Source: CAD feature listing. Evaluate the final solid. Frame: model axes, mm. Face numbers are marked on the shaded views. Give positions to 0.01 mm unless a question says otherwise; leave off trailing zeros. Write each loop counter-clockwise with the first axis right and the second up, starting at its lowest first coordinate (ties: lowest second). Pieces come first, ordered by that corner, then holes. Notation, with made-up numbers: (-36, -22) -> (-23, -22) arc R10 cw to (-23, -6) -> close; hole circle Ø3 at (26.5, 12). An arc over 180 degrees is marked (long way). Write item = value, one per line.
from build123d import *

# Parameters (mm, degrees)
F0_W     = 6
F0_H     = 25
F0_W_2   = 5
F0_W_3   = 12.7
F0_H_2   = 10
F0_H_3   = 5
F0_W_4   = 6.15
F1_DEPTH = 3
F0_W_5   = 10
F2_DEPTH = 3.25


with BuildPart() as f1:
    # F0 (on Top) → F1 (new body)
    with BuildSketch(Plane.XY):
        with Locations((-39.9078816451, 39.8015151515)):
            Rectangle(F0_W, F0_H)
        Polygon((-11.9078816451, 27.3015151515), (0.5921183549, 27.3015151515), (0.5921183549, 52.3015151515), (-36.9078816451, 52.3015151515), (-36.9078816451, 27.3015151515), align=None)
        Polygon((0.5921183549, 27.3015151515), (13.0921183549, 27.3015151515), (39.0921183549, 27.3015151515), (39.0921183549, 52.3015151515), (0.5921183549, 52.3015151515), align=None)
        with Locations((41.5921183549, 39.8015151515)):
            Rectangle(F0_W_2, F0_H)
        with Locations((0.5921183549, -99.7984848485)):
            Rectangle(F0_W_3, F0_H_2)
        with Locations((0.5921183549, -92.2984848485)):
            Rectangle(F0_W_3, F0_H_3)
        with Locations((10.0171183549, -92.2984848485)):
            Rectangle(F0_W_4, F0_H_3)
        Polygon((6.9421183549, -89.7984848485), (13.0921183549, -89.7984848485), (13.0921183549, 27.3015151515), (0.5921183549, 27.3015151515), (-11.9078816451, 27.3015151515), (-11.9078816451, -89.7984848485), (-5.7578816451, -89.7984848485), align=None)
        with Locations((-8.8328816451, -92.2984848485)):
            Rectangle(F0_W_4, F0_H_3)
    extrude(amount=F1_DEPTH)

    # F0 (on Top) → F2 (join)
    with BuildSketch(Plane.XY):
        with Locations((10.0171183549, -99.7984848485)):
            Rectangle(F0_W_4, F0_H_2)
        with Locations((-8.8328816451, -99.7984848485)):
            Rectangle(F0_W_4, F0_H_2)
        with Locations((-47.9078816451, 39.8015151515)):
            Rectangle(F0_W_5, F0_H)
        with Locations((49.0921183549, 39.8015151515)):
            Rectangle(F0_W_5, F0_H)
    extrude(amount=F2_DEPTH)


solid = f1.part
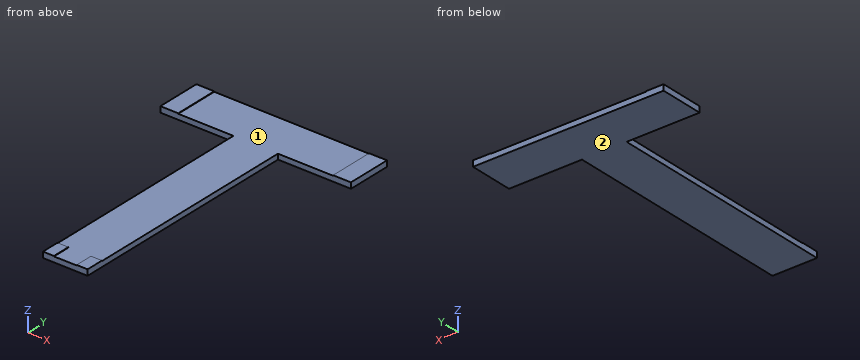
1) Cut plane D-D (x = 25). Return the cut outline in (y, z), then the cut area to 3 significant figures.
Computed:
outline = (27.3, 0) -> (52.3, 0) -> (52.3, 3) -> (27.3, 3) -> close
area = 75.0 mm²
2) Material intervals for L1, parallel to X at y = -51, z = 2.6; L2, parallel to Y at x = -47.5, z = 1.2; L3, parallel to Z at x = -33, y = 42, sorted ascending.
Computed:
L1 = -11.91 to 13.09
L2 = 27.3 to 52.3
L3 = 0 to 3
3) Cut plane B-B (y = 35). Return the cut outline in (x, z), then the cut area to 3 significant figures.
Computed:
outline = (-52.91, 0) -> (54.09, 0) -> (54.09, 3.25) -> (44.09, 3.25) -> (44.09, 3) -> (-42.91, 3) -> (-42.91, 3.25) -> (-52.91, 3.25) -> close
area = 326 mm²
4) Contact query for flat-ended pins moving along their axis: pin 1 (1 mm diameter, centred on y = -55, z = 1, fed in from +X); pin 2 (1 mm diameter, centred on y = 8.5, z = 1, fed in from -X); pin 3 (3 mm diameter, centred on x = -7.5, y = -2.5, fed in from +Z). Output: stop coordinate, or through.
Computed:
pin_1 = 13.09
pin_2 = -11.91
pin_3 = 3
5) Cut plane A-A (x = 9.5). Return the cut outline in (y, z), then the cut area to 3 significant figures.
Computed:
outline = (-104.8, 0) -> (52.3, 0) -> (52.3, 3) -> (-94.8, 3) -> (-94.8, 3.25) -> (-104.8, 3.25) -> close
area = 474 mm²
6) Draft query along X for the marked faces 1 and 2. Return one class per face: pulls with the +X half, pulls with the -X half, needs draft (parallel to the pull), parting line crosses it, or undercut.
Computed:
face_1 = undercut
face_2 = needs draft
7) Cut plane C-C (z = 1.7). Return the cut outline in (x, y).
Computed:
outline = (-52.91, 27.3) -> (-11.91, 27.3) -> (-11.91, -104.8) -> (13.09, -104.8) -> (13.09, 27.3) -> (54.09, 27.3) -> (54.09, 52.3) -> (-52.91, 52.3) -> close
